from build123d import *

# Parameters (mm, degrees)
BOSS_EXTRUDE3_DEPTH = 2.5
BOSS_EXTRUDE4_DEPTH = 29
SKETCH4_W           = 2.589054973
SKETCH4_H           = 105.965654802
SKETCH4_W_2         = 105.965002317
SKETCH4_H_2         = 1.925754282
BOSS_EXTRUDE5_DEPTH = 18


with BuildPart() as part:
    # Sketch1 → Revolve1 (revolve)
    with BuildSketch(Plane.YZ, mode=Mode.PRIVATE) as revolve1_sk:
        with BuildLine():
            Line((0, 45), (25, 45))
            Line((25, 45), (25, 53))
            ThreePointArc((25, 53), (12.5, 57), (0, 53))
            Line((0, 53), (0, 45))
        make_face()
    revolve(revolve1_sk.sketch.rotate(Axis((0, 0, 0), (0, 1, 0)), 180), axis=Axis((0, 0, 0), (0, 1, 0)))

    # Sketch2 → Boss-Extrude3 (add)
    with BuildSketch(Plane(origin=(0, 25, 0), x_dir=(-1, 0, 0), z_dir=(0, 1, 0))):
        with BuildLine():
            Line((42.797543233, 13.905764747), (0, 0))
            Line((0, 0), (0, 44.974993052))
            Line((0, 44.974993052), (0, 45))
            ThreePointArc((0, 45), (-0.750104217, 44.993747829), (-1.5, 44.974993052))
            Line((-1.5, 44.974993052), (-6.465637775, 8.899186938))
            Line((-6.465637775, 8.899186938), (-42.310234721, 15.324621949))
            ThreePointArc((-42.310234721, 15.324621949), (-42.797543233, 13.905764747), (-43.237285704, 12.4714524))
            Line((-43.237285704, 12.4714524), (-10.461621679, -3.399186938))
            Line((-10.461621679, -3.399186938), (-27.649163129, -35.503855822))
            ThreePointArc((-27.649163129, -35.503855822), (-26.450336353, -36.405764747), (-25.222112146, -37.267211579))
            Line((-25.222112146, -37.267211579), (0, -11))
            Line((0, -11), (25.222112146, -37.267211579))
            ThreePointArc((25.222112146, -37.267211579), (26.450336353, -36.405764747), (27.649163129, -35.503855822))
            Line((27.649163129, -35.503855822), (10.461621679, -3.399186938))
            Line((10.461621679, -3.399186938), (43.237285704, 12.4714524))
            ThreePointArc((43.237285704, 12.4714524), (43.023392016, 13.190441216), (42.797543233, 13.905764747))
        make_face()
        with BuildLine():
            Line((6.465637775, 8.899186938), (0, 0))
            Line((0, 0), (42.797543233, 13.905764747))
            ThreePointArc((42.797543233, 13.905764747), (42.559802114, 14.617224223), (42.310234721, 15.324621949))
            Line((42.310234721, 15.324621949), (6.465637775, 8.899186938))
        make_face()
        Polygon((0, 44.974993052), (0, 0), (6.465637775, 8.899186938), (1.5, 44.974993052), align=None)
        with BuildLine():
            Line((0, 45), (0, 44.974993052))
            Line((0, 44.974993052), (1.5, 44.974993052))
            ThreePointArc((1.5, 44.974993052), (0.750104217, 44.993747829), (0, 45))
        make_face()
    extrude(amount=-BOSS_EXTRUDE3_DEPTH)

    # Sketch3 → Boss-Extrude4 (add)
    with BuildSketch(Plane.XZ.offset(-22.5)):
        with BuildLine():
            Line((1.75, 4.145780988), (1.75, 2.436698586))
            ThreePointArc((1.75, 2.436698586), (2.669269563, 1.369306394), (3, 0))
            ThreePointArc((3, 0), (2.669269563, -1.369306394), (1.75, -2.436698586))
            Line((1.75, -2.436698586), (1.75, -4.145780988))
            ThreePointArc((1.75, -4.145780988), (3.75, -2.487468593), (4.5, 0))
            ThreePointArc((4.5, 0), (3.75, 2.487468593), (1.75, 4.145780988))
        make_face()
        with BuildLine():
            ThreePointArc((3, 0), (2.669269563, 1.369306394), (1.75, 2.436698586))
            Line((1.75, 2.436698586), (1.75, 0))
            Line((1.75, 0), (1.75, -2.436698586))
            ThreePointArc((1.75, -2.436698586), (2.669269563, -1.369306394), (3, 0))
        make_face()
        with BuildLine():
            Line((-1.75, -2.436698586), (-1.75, 0))
            Line((-1.75, 0), (-1.75, 2.436698586))
            ThreePointArc((-1.75, 2.436698586), (-3, 0), (-1.75, -2.436698586))
        make_face()
        with BuildLine():
            ThreePointArc((-1.75, -2.436698586), (-3, 0), (-1.75, 2.436698586))
            Line((-1.75, 2.436698586), (-1.75, 4.145780988))
            ThreePointArc((-1.75, 4.145780988), (-4.5, 0), (-1.75, -4.145780988))
            Line((-1.75, -4.145780988), (-1.75, -2.436698586))
        make_face()
        with BuildLine():
            Line((-1.75, 4.145780988), (-1.75, 2.436698586))
            ThreePointArc((-1.75, 2.436698586), (0, 3), (1.75, 2.436698586))
            Line((1.75, 2.436698586), (1.75, 4.145780988))
            ThreePointArc((1.75, 4.145780988), (0, 4.5), (-1.75, 4.145780988))
        make_face()
        with BuildLine():
            ThreePointArc((1.75, -2.436698586), (0, -3), (-1.75, -2.436698586))
            Line((-1.75, -2.436698586), (-1.75, -4.145780988))
            ThreePointArc((-1.75, -4.145780988), (0, -4.5), (1.75, -4.145780988))
            Line((1.75, -4.145780988), (1.75, -2.436698586))
        make_face()
    extrude(amount=BOSS_EXTRUDE4_DEPTH)

    # Sketch4 → Boss-Extrude5 (add)
    with BuildSketch(Plane(origin=(0, 25, 0), x_dir=(-1, 0, 0), z_dir=(0, 1, 0))):
        with Locations((0.379622384, 0.0092753)):
            Rectangle(SKETCH4_W, SKETCH4_H)
        with Locations((0.017498841, -0.962877141)):
            Rectangle(SKETCH4_W_2, SKETCH4_H_2)
    extrude(amount=BOSS_EXTRUDE5_DEPTH)


solid = part.part
Geometry check sheet. Reference: the model listing, model coordinates, mm. A direction names the side the tool comes from. Give positions to 0.01 mm unless a question says otherwise; leave off trailing zeros. Write each loop counter-clockwise with the first axis right and the second up, starting at its lowest first coordinate (ties: lowest second). Pieces come first, ordered by that corner, then holes. Notation, with made-up numbers: (34.5, -38) - (77.5, -38) arc R24 cw to (77.5, -1) - close; hole circle Ø3 at (-23, 73.5). An arc over 180 degrees is marked (long way). Put each result on its own line as item: value.
1. Thickness scan on line 1 (X direction, y = 12, z = 0); line 2 (X direction, y = 16, z = 0); line 3 (Z direction, x = -33, y = 24.5). Record the ranges inside material, lowest first.
Ans:
line 1: x = -56.99 to -45, -4.5 to -1.75, 1.75 to 4.5, 45 to 56.99
line 2: x = -56.71 to -45, -4.5 to -1.75, 1.75 to 4.5, 45 to 56.71
line 3: z = -41.91 to -30.59, 7.51 to 13.66, 30.59 to 41.91
2. Draft check along Z on faces 1 (the flat face through (0, 34, 52.992)), 2 (the flat face through (-26.62, 23.768, 4.425)), 3 (the flat face through (-1.674, 34, -28)). Enter one of: +Z half, -Z half, draft (parallel to the pull), parting line (faces both ways), or undercut.
Ans:
face 1: +Z half
face 2: undercut
face 3: draft
3. Go/stop test with flat-tipped pins: pin 1 (2 mm diameter, centred on x = -0.5, y = 37, fed in from +Z); pin 2 (1 mm diameter, centred on y = 17.5, z = 32, fed in from -X); pin 3 (14.5 mm diameter, centred on y = 35, z = -39.5, fed in from -X); pin 4 (8 mm diameter, centred on x = 30, z = -7.5, fed in from +Y). Record where each tip stops, or that it passes through.
Ans:
pin 1: stops at z = 52.99
pin 2: stops at x = -46.83
pin 3: stops at x = -1.67
pin 4: passes through
4. Sectioned sample at A-A, the plane y = 14. Enter the section's corners in (x, z), plus the area to 3 significant figures.
Ans:
outline: circle Ø113.9 at (0, 0); circle Ø9 at (0, 0); hole circle Ø90 at (0, 0); hole (-1.75, -2.44) arc R3 ccw to (1.75, -2.44) - (1.75, 2.44) arc R3 ccw to (-1.75, 2.44) - close
area: 3,870 mm²
5. Sectioned sample at B-B, the plane x = -39. Give the number of separate pieces and of enclosed holes in the cut face, plus the area to 3 significant figures.
Ans:
separate pieces: 4
enclosed holes: 0
area: 912 mm²
6. Set-up check for faces 4 (the flat face through (0.915, 34, -28)), 5 (the flat face through (-27, 34, 0)), 6 (the flat face through (24.137, 23.768, 12.067)): record each of +Z, -Z, +X, -X, +Y, -Y from which the full face is reachable in a straight line by a thin tool's end or side.
Ans:
face 4: -Z, +X, +Y
face 5: +Z, -X, +Y
face 6: +Y, -Y
